Verification items for the finished model (mm, model axes). Face numbers are marked on the shaded views. A direction names the side the tool comes from. Round coordinates to 2 decimals unless told otherwise and drop trailing zeros. Order: outer loops, then holes, each group sorted by start corner. A loop starts at its lowest first (then second) coordinate and runs counter-clockwise, first axis right, second up. Notation, with made-up numbers: (77, 83.5) -> (85, 83.5) arc R26 ccw to (85, 97.5) -> close; hole circle Ø7 at (15.5, 50.25). An arc over 180 degrees is marked (long way). Answer in a Markdown table with one row per item. Add a question column.
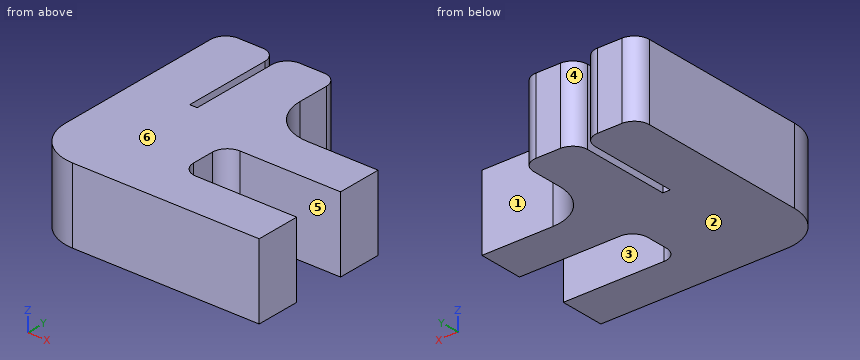
```python
from build123d import *

# Parameters (mm, degrees)
F1_DEPTH = 5


with BuildPart() as f1:
    # F0 (on Top) → F1 (new body)
    with BuildSketch(Plane.XY):
        with BuildLine():
            Line((-34.368042, 42.236285), (-35.993042, 42.236285))
            ThreePointArc((-35.993042, 42.236285), (-36.700148, 41.943392), (-36.993042, 41.236285))
            Line((-36.993042, 41.236285), (-36.993042, 29.636285))
            ThreePointArc((-36.993042, 29.636285), (-36.114362, 27.514965), (-33.993042, 26.636285))
            Line((-33.993042, 26.636285), (-21.493042, 26.636285))
            Line((-21.493042, 26.636285), (-21.493042, 29.636285))
            Line((-21.493042, 29.636285), (-28.243042, 29.636285))
            ThreePointArc((-28.243042, 29.636285), (-28.950148, 29.929179), (-29.243042, 30.636285))
            Line((-29.243042, 30.636285), (-29.243042, 32.136285))
            ThreePointArc((-29.243042, 32.136285), (-28.950148, 32.843392), (-28.243042, 33.136285))
            Line((-28.243042, 33.136285), (-21.493042, 33.136285))
            Line((-21.493042, 33.136285), (-21.493042, 36.136285))
            Line((-21.493042, 36.136285), (-26.243042, 36.136285))
            ThreePointArc((-26.243042, 36.136285), (-28.364362, 37.014965), (-29.243042, 39.136285))
            Line((-29.243042, 39.136285), (-29.243042, 41.236285))
            ThreePointArc((-29.243042, 41.236285), (-29.535935, 41.943392), (-30.243042, 42.236285))
            Line((-30.243042, 42.236285), (-31.868042, 42.236285))
            ThreePointArc((-31.868042, 42.236285), (-32.575148, 41.943392), (-32.868042, 41.236285))
            Line((-32.868042, 41.236285), (-32.868042, 35.236285))
            Line((-32.868042, 35.236285), (-33.368042, 35.236285))
            Line((-33.368042, 35.236285), (-33.368042, 41.236285))
            ThreePointArc((-33.368042, 41.236285), (-33.660935, 41.943392), (-34.368042, 42.236285))
        make_face()
    extrude(amount=F1_DEPTH)


solid = f1.part
```
1) Cross-section at D-D, the plane y = 28.25. Record the boundary of the cut face in (x, z).
2) Cross-section at C-C, the plane z = 4.1. Record the boundary of the cut face in (x, y), and give its area (3 significant figures).
3) Tool access check on the marked faces 1, 2 and 3. Record the directions out of +Z, -Z, +X, -X, +Y, -Y that give a thin tool (end or side, any length) a straight path to the whole face; none if there is none.
4) Thickness scan on L1, parallel to X at y = 39, z = 4.65; L2, parallel to Y at x = -23, z = 0.7; L3, parallel to X at y = 31.25, z = 0.4. Record the ranges inside material, lowest first. Write a range as [from, to].
5) Depth check by flat-ended pin: P1, Ø2.5, axis at x = -24.5, z = 1.5, coming from the +Y side; P2, Ø1, axis at x = -35, z = 0.5, coming from the -Y side; P3, Ø1.1, axis at y = 40.5, z = 2, coming from the +X side. Enter the tip coordinate at first touch or a pass-through.
6) Cross-section at B-B, the plane x = -27.5. Record the boundary of the cut face in (y, z), and give its area (3 significant figures).
7) Cross-section at A-A, the plane y = 35.5. Record the boundary of the cut face in (x, z).
8) Draft check along Y on the marked faces 4, 5 and 6. Enter one of: +Y half, -Y half, draft (parallel to the pull), parting line (faces both ways), or undercut.
Results below:
| question | item | result |
|---|---|---|
| 1 | outline | (-36.65, 0) -> (-21.49, 0) -> (-21.49, 5) -> (-36.65, 5) -> close |
| 2 | outline | (-36.99, 29.64) arc R3 ccw to (-33.99, 26.64) -> (-21.49, 26.64) -> (-21.49, 29.64) -> (-28.24, 29.64) arc R1 cw to (-29.24, 30.64) -> (-29.24, 32.14) arc R1 cw to (-28.24, 33.14) -> (-21.49, 33.14) -> (-21.49, 36.14) -> (-26.24, 36.14) arc R3 cw to (-29.24, 39.14) -> (-29.24, 41.24) arc R1 ccw to (-30.24, 42.24) -> (-31.87, 42.24) arc R1 ccw to (-32.87, 41.24) -> (-32.87, 35.24) -> (-33.37, 35.24) -> (-33.37, 41.24) arc R1 ccw to (-34.37, 42.24) -> (-35.99, 42.24) arc R1 ccw to (-36.99, 41.24) -> close |
| 2 | area | 163 mm² |
| 3 | face 1 | +Z, -Z, +X, +Y |
| 3 | face 2 | -Z, +X, -X, +Y, -Y |
| 3 | face 3 | +Z, -Z, +X |
| 4 | L1 | [-36.99, -33.37], [-32.87, -29.24] |
| 4 | L2 | [26.64, 29.64], [33.14, 36.14] |
| 4 | L3 | [-36.99, -29.24] |
| 5 | P1 | y = 36.14 |
| 5 | P2 | y = 26.68 |
| 5 | P3 | x = -29.24 |
| 6 | outline | (26.64, 0) -> (29.64, 0) -> (29.64, 5) -> (26.64, 5) -> close; (33.14, 0) -> (36.41, 0) -> (36.41, 5) -> (33.14, 5) -> close |
| 6 | area | 31.4 mm² |
| 7 | outline | (-36.99, 0) -> (-33.37, 0) -> (-33.37, 5) -> (-36.99, 5) -> close; (-32.87, 0) -> (-21.49, 0) -> (-21.49, 5) -> (-32.87, 5) -> close |
| 8 | face 4 | +Y half |
| 8 | face 5 | undercut |
| 8 | face 6 | draft |
